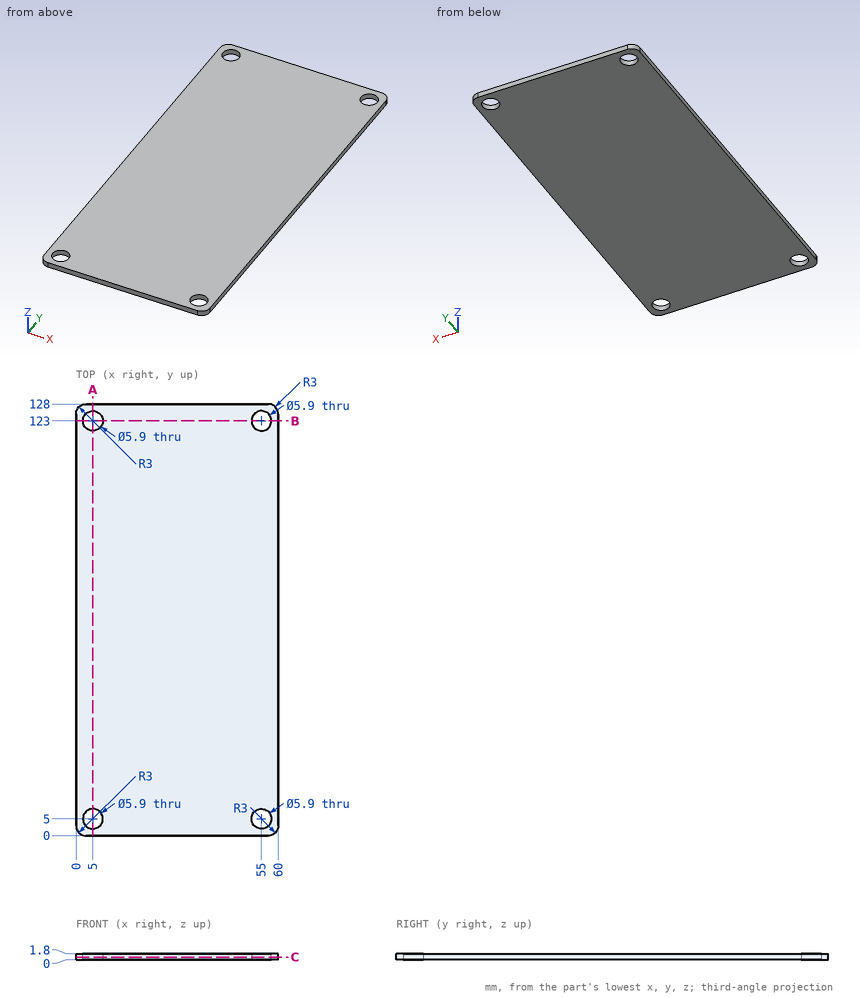
Print and shaded views of the part. All mm, measured from the part's lowest x, y and z. Give positions to 0.01 mm unless a question says otherwise; leave off trailing zeros. Write each loop counter-clockwise with the first axis right and the second up, starting at its lowest first coordinate (ties: lowest second). Pieces come first, ordered by that corner, then holes. Notation, with made-up numbers: (79, 9.25) -> (135, 9.25) arc R28 cw to (135, 43.25) -> close; hole circle Ø4 at (-21.5, -10.5). An arc over 180 degrees is marked (long way). Write each question's results on one line, items separated by ' | '.
1. Cut at A-A, the plane x = 5. Write the cut outline in (y, z), then the cut area to 3 significant figures.
Geometry check:
outline: (0, 0) -> (2.05, 0) -> (2.05, 1.8) -> (0, 1.8) -> close; (7.95, 0) -> (120.05, 0) -> (120.05, 1.8) -> (7.95, 1.8) -> close; (125.95, 0) -> (128, 0) -> (128, 1.8) -> (125.95, 1.8) -> close | area: 209 mm²
2. Cut at B-B, the plane y = 123. Write the cut outline in (x, z), then the cut area to 3 significant figures.
Geometry check:
outline: (0, 0) -> (2.05, 0) -> (2.05, 1.8) -> (0, 1.8) -> close; (7.95, 0) -> (52.05, 0) -> (52.05, 1.8) -> (7.95, 1.8) -> close; (57.95, 0) -> (60, 0) -> (60, 1.8) -> (57.95, 1.8) -> close | area: 86.8 mm²
3. Wall check: probe 1 along Y at (x, z) = (5, 1.2); probe 2 along X at (y, z) = (5, 0.95). Give the ranges that are in metal, low to high. Write a range as [from, to].
Geometry check:
probe 1: [0, 2.05], [7.95, 120.05], [125.95, 128] | probe 2: [0, 2.05], [7.95, 52.05], [57.95, 60]
4. Cut at C-C, the plane z = 0.8. Write the cut outline in (x, y).
Geometry check:
outline: (0, 3) arc R3 ccw to (3, 0) -> (57, 0) arc R3 ccw to (60, 3) -> (60, 125) arc R3 ccw to (57, 128) -> (3, 128) arc R3 ccw to (0, 125) -> close; hole circle Ø5.9 at (5, 5); hole circle Ø5.9 at (5, 123); hole circle Ø5.9 at (55, 5); hole circle Ø5.9 at (55, 123)
5. Drop flat-ended pins along their axis: P1, Ø4.5, axis at x = 5, y = 123, coming from the +Z side; P2, Ø12, axis at x = 12, y = 48.5, coming from the -Z side. Give the stop position or say it passes through.
Geometry check:
P1: through | P2: z = 0
